CAD build for the part. Positions are in the model's coordinates, mm. Face numbers are marked on the shaded views. A direction names the side the tool comes from. Round coordinates to 2 decimals unless told otherwise and drop trailing zeros. Loops run counter-clockwise (first coordinate to the right, second up) from the corner with the lowest first, then second, coordinate; pieces in that order, holes last.
```python
from build123d import *

# Parameters (mm, degrees)
F0_W     = 22.5
F0_H     = 9
F1_DEPTH = 5.5
F2_R     = 3
F3_DEPTH = 3.25
F4_R     = 1.6
F5_DEPTH = 2.5
F6_R     = 4.49999
F7_R     = 2
F8_R     = 1.49999


# Not quite as in the source:
# - a fillet or chamfer is up to 0.001 mm smaller than in the source, because OpenCascade refuses the exact size


with BuildPart() as f1:
    # F0 (on Top) → F1 (new body)
    with BuildSketch(Plane.XY):
        with Locations((-6.75, 0)):
            Rectangle(F0_W, F0_H)
    extrude(amount=F1_DEPTH)

    # F2 (on face) → F3 (cut)
    with BuildSketch(Plane.XY.offset(5.5)):
        Circle(F2_R)
    extrude(amount=-F3_DEPTH, mode=Mode.SUBTRACT)

    # F4 (on face) → F5 (cut)
    with BuildSketch(Plane.XY.offset(2.25)):
        Circle(F4_R)
    extrude(amount=-F5_DEPTH, mode=Mode.SUBTRACT)

    # F6 (radius 4.5 in the source; OpenCascade refuses exactly that, so slightly less here)
    f6_edges = [f1.edges().sort_by_distance(p)[0] for p in [
        (4.5, -4.5, 2.75),
        (4.5, 4.5, 2.75),
    ]]
    fillet(f6_edges, radius=F6_R)

    # F7
    f7_edges = [f1.edges().sort_by_distance(p)[0] for p in [
        (-18, 4.5, 2.75),
        (-18, -4.5, 2.75),
    ]]
    fillet(f7_edges, radius=F7_R)

    # F8 (radius 1.5 in the source; OpenCascade refuses exactly that, so slightly less here)
    f8_edges = [f1.edges().sort_by_distance(p)[0] for p in [
        (-7.999995, -4.5, 5.5),
    ]]
    fillet(f8_edges, radius=F8_R)


solid = f1.part
```
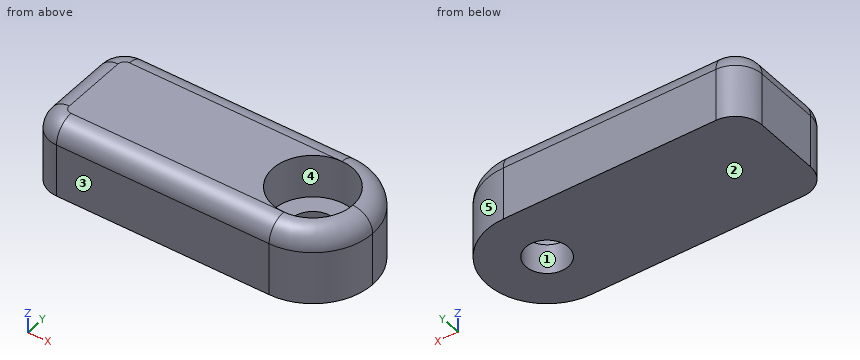
Item 1: 3-axis set-ups, long thin cutter, end or side, ignore diameter. For the marked faces 4 and 5: which of +Z, -Z, +X, -X, +Y, -Y reach the whole face in a straight line?
Answers follow:
face 4: +Z
face 5: +Z, -Z, +X, +Y
Item 2: Flat gauge pins, fed straight in: P1, Ø4, axis at x = -10.5, y = 3.5, coming from the -Z side; P2, Ø3, axis at x = 0, y = -1, coming from the +Z side. Where does each tip first touch, or does it go through?
Answers follow:
P1: stops at z = 0
P2: stops at z = 2.25
Item 3: Probe line 1 (Y direction, x = 0, z = 1.25); line 2 (Y direction, x = 0, z = 3.5); line 3 (X direction, y = -0.5, z = 1.2). List the from-to ranges inside material, lowest first.
Answers follow:
line 1: y = -4.5 to -1.6, 1.6 to 4.5
line 2: y = -4.5 to -3, 3 to 4.5
line 3: x = -18 to -1.52, 1.52 to 4.47
Item 4: Cut at D-D, the plane x = -2.25. Give the cut face in (y, z), plus the area to 3 significant figures.
Answers follow:
outline: (-4.5, 0) - (4.5, 0) - (4.5, 4) arc R1.5 ccw to (3, 5.5) - (1.98, 5.5) - (1.98, 2.25) - (-1.98, 2.25) - (-1.98, 5.5) - (-3, 5.5) arc R1.5 ccw to (-4.5, 4) - close
area: 35.6 mm2
Item 5: Cut at B-B, the plane x = -11.5. Give the cut face in (y, z), plus the area to 3 significant figures.
Answers follow:
outline: (-4.5, 0) - (4.5, 0) - (4.5, 4) arc R1.5 ccw to (3, 5.5) - (-3, 5.5) arc R1.5 ccw to (-4.5, 4) - close
area: 48.5 mm2
Item 6: Two-plate mould, pull along Y, no slides. Class the marked faces 1, 2 and 3: released by +Y, released by -Y, zero draft, split by the parting line, or undercut.
Answers follow:
face 1: undercut
face 2: zero draft
face 3: released by -Y
